The listing builds one solid part. Answer for the finished solid, in the listing's coordinates (mm). Coordinates: 2 decimals unless noted, no trailing zeros. Loops run counter-clockwise (first coordinate to the right, second up) from the corner with the lowest first, then second, coordinate; pieces in that order, holes last. Notation, with made-up numbers: (-29.75, 23) - (3.25, 23) arc R26 cw to (3.25, 52) - close; hole circle Ø2 at (52.25, 40.5). An arc over 180 degrees is marked (long way). One line per question, with ' | ' between items.
from build123d import *

# Parameters (mm, degrees)
F0_R     = 1.5875
F1_DEPTH = 3.048


with BuildPart() as f1:
    # F0 (on Front) → F1 (new body)
    with BuildSketch(Plane.XZ):
        with BuildLine():
            ThreePointArc((-9.5341186691, 52.2447508267), (-6.7171678622, 45.5597172954), (-0.0094340062, 42.7972561321))
            ThreePointArc((-0.0094340062, 42.7972561321), (6.7257580846, 45.5870640413), (9.5155659938, 52.3222561321))
            ThreePointArc((9.5155659938, 52.3222561321), (9.4949130682, 52.9491625761), (9.4330438542, 53.573350395))
            ThreePointArc((9.4330438542, 53.573350395), (0.5455224312, 61.8310756357), (-9.2422673958, 54.6632842395))
            Line((-9.2422673958, 54.6632842395), (-9.5341186691, 52.2447508267))
        make_face()
        with BuildLine():
            ThreePointArc((3.1655659938, 52.3222561321), (2.235630024, 50.0771921018), (-0.0094340062, 49.1472561321))
            ThreePointArc((-0.0094340062, 49.1472561321), (-2.2544980365, 54.5673201623), (3.1655659938, 52.3222561321))
        make_face(mode=Mode.SUBTRACT)
        with BuildLine():
            ThreePointArc((9.5155659938, 52.3222561321), (6.7257580846, 45.5870640413), (-0.0094340062, 42.7972561321))
            Line((-0.0094340062, 42.7972561321), (-0.0094340062, 38.0458299899))
            Line((-0.0094340062, 38.0458299899), (0.1854236079, 17.3965493596))
            ThreePointArc((0.1854236079, 17.3965493596), (10.4432233162, 13.7633317509), (15.9512497798, 4.3780043978))
            Line((15.9512497798, 4.3780043978), (9.4330438542, 53.573350395))
            ThreePointArc((9.4330438542, 53.573350395), (9.4949130682, 52.9491625761), (9.5155659938, 52.3222561321))
        make_face()
        with BuildLine():
            Line((-0.0094340062, 38.0458299899), (-0.0094340062, 42.7972561321))
            ThreePointArc((-0.0094340062, 42.7972561321), (-6.7171678622, 45.5597172954), (-9.5341186691, 52.2447508267))
            Line((-9.5341186691, 52.2447508267), (-15.4254400006, 3.4241398184))
            ThreePointArc((-15.4254400006, 3.4241398184), (-10.3245703873, 13.2859483017), (-0.0094340062, 17.3935143465))
            Line((-0.0094340062, 17.3935143465), (-0.0094340062, 38.0458299899))
        make_face()
        with Locations((-1.6167838335, 40.1418484393)):
            Circle(F0_R, mode=Mode.SUBTRACT)
        with BuildLine():
            ThreePointArc((-9.2422673958, 54.6632842395), (-9.4658311447, 53.4633863439), (-9.5341186691, 52.2447508267))
            Line((-9.5341186691, 52.2447508267), (-9.2422673958, 54.6632842395))
        make_face()
        with BuildLine():
            Line((-0.0094340062, 4.678493973), (-0.0094340062, 17.3935143465))
            ThreePointArc((-0.0094340062, 17.3935143465), (-10.3245703873, 13.2859483017), (-15.4254400006, 3.4241398184))
            ThreePointArc((-15.4254400006, 3.4241398184), (-15.5386299257, 1.7131836533), (-15.4666248709, 0))
            ThreePointArc((-15.4666248709, 0), (-10.4652805135, -10.1123806344), (-0.0094340062, -14.3490020823))
            Line((-0.0094340062, -14.3490020823), (-0.0094340062, -1.6339817089))
            ThreePointArc((-0.0094340062, -1.6339817089), (-2.8397781032, 1.5222561321), (-0.0094340062, 4.678493973))
        make_face()
        with BuildLine():
            ThreePointArc((15.9512497798, 4.3780043978), (10.4432233162, 13.7633317509), (0.1854236079, 17.3965493596))
            Line((0.1854236079, 17.3965493596), (0.305262239, 4.6971147776))
            ThreePointArc((0.305262239, 4.6971147776), (2.5696684822, 3.7778876305), (3.5102218968, 1.5222561321))
            ThreePointArc((3.5102218968, 1.5222561321), (2.4549320784, -0.8415234148), (-0.0094340062, -1.6339817089))
            Line((-0.0094340062, -1.6339817089), (-0.0094340062, -14.3490020823))
            ThreePointArc((-0.0094340062, -14.3490020823), (8.4967936253, -12.09407127), (14.495092683, -5.6550472833))
            ThreePointArc((14.495092683, -5.6550472833), (15.7754870132, -2.1674373693), (16.2102218968, 1.5222561321))
            ThreePointArc((16.2102218968, 1.5222561321), (16.1453463055, 2.9559894332), (15.9512497798, 4.3780043978))
        make_face()
        with BuildLine():
            ThreePointArc((-0.0094340062, -14.3490020823), (-10.4652805135, -10.1123806344), (-15.4666248709, 0))
            Line((-15.4666248709, 0), (-9.5284841955, -61.6411305964))
            ThreePointArc((-9.5284841955, -61.6411305964), (-6.6245448741, -55.1245742942), (-0.0094340062, -52.4527438679))
            Line((-0.0094340062, -52.4527438679), (-0.0094340062, -14.3490020823))
        make_face()
        with BuildLine():
            ThreePointArc((14.495092683, -5.6550472833), (8.4967936253, -12.09407127), (-0.0094340062, -14.3490020823))
            Line((-0.0094340062, -14.3490020823), (-0.0094340062, -52.4527438679))
            ThreePointArc((-0.0094340062, -52.4527438679), (6.7257580846, -55.2425517771), (9.5155659938, -61.9777438679))
            Line((9.5155659938, -61.9777438679), (36.5030659938, -61.9777438679))
            ThreePointArc((36.5030659938, -61.9777438679), (38.9286766306, -56.2660907011), (44.7230299367, -54.0452713422))
            Line((44.7230299367, -54.0452713422), (18.5079615272, -53.1084211888))
            ThreePointArc((18.5079615272, -53.1084211888), (12.8201303591, -50.41150042), (10.8761098535, -44.4243818055))
            Line((10.8761098535, -44.4243818055), (14.495092683, -5.6550472833))
        make_face()
        with BuildLine():
            ThreePointArc((-0.0094340062, -52.4527438679), (-6.6245448741, -55.1245742942), (-9.5284841955, -61.6411305964))
            ThreePointArc((-9.5284841955, -61.6411305964), (-6.8593267813, -68.5962477752), (0, -71.502739196))
            Line((0, -71.502739196), (0.6586396335, -71.4792859855))
            ThreePointArc((0.6586396335, -71.4792859855), (6.9579552616, -68.4724426131), (9.5155659938, -61.9777438679))
            Line((9.5155659938, -61.9777438679), (3.1655659938, -61.9777438679))
            ThreePointArc((3.1655659938, -61.9777438679), (-2.2544980365, -64.2228078982), (-0.0094340062, -58.8027438679))
            Line((-0.0094340062, -58.8027438679), (-0.0094340062, -52.4527438679))
        make_face()
        with BuildLine():
            Line((0.6586396335, -71.4792859855), (0, -71.502739196))
            ThreePointArc((0, -71.502739196), (0.3295227253, -71.4967108988), (0.6586396335, -71.4792859855))
        make_face()
        with BuildLine():
            Line((36.5030659938, -61.9777438679), (9.5155659938, -61.9777438679))
            ThreePointArc((9.5155659938, -61.9777438679), (6.9579552616, -68.4724426131), (0.6586396335, -71.4792859855))
            Line((0.6586396335, -71.4792859855), (44.7230299367, -69.9102163936))
            ThreePointArc((44.7230299367, -69.9102163936), (38.9286766306, -67.6893970348), (36.5030659938, -61.9777438679))
        make_face()
        with BuildLine():
            ThreePointArc((44.7230299367, -54.0452713422), (38.9286766306, -56.2660907011), (36.5030659938, -61.9777438679))
            ThreePointArc((36.5030659938, -61.9777438679), (38.9286766306, -67.6893970348), (44.7230299367, -69.9102163936))
            ThreePointArc((44.7230299367, -69.9102163936), (50.1522191606, -67.4896332311), (52.3780659938, -61.9777438679))
            ThreePointArc((52.3780659938, -61.9777438679), (50.1522191606, -56.4658545048), (44.7230299367, -54.0452713422))
        make_face()
        with BuildLine():
            ThreePointArc((47.6155659938, -61.9777438679), (44.4405659938, -65.1527438679), (41.2655659938, -61.9777438679))
            ThreePointArc((41.2655659938, -61.9777438679), (44.4405659938, -58.8027438679), (47.6155659938, -61.9777438679))
        make_face(mode=Mode.SUBTRACT)
        with BuildLine():
            ThreePointArc((9.5155659938, -61.9777438679), (6.7257580846, -55.2425517771), (-0.0094340062, -52.4527438679))
            Line((-0.0094340062, -52.4527438679), (-0.0094340062, -58.8027438679))
            ThreePointArc((-0.0094340062, -58.8027438679), (2.235630024, -59.7326798377), (3.1655659938, -61.9777438679))
            Line((3.1655659938, -61.9777438679), (9.5155659938, -61.9777438679))
        make_face()
    extrude(amount=F1_DEPTH)


solid = f1.part
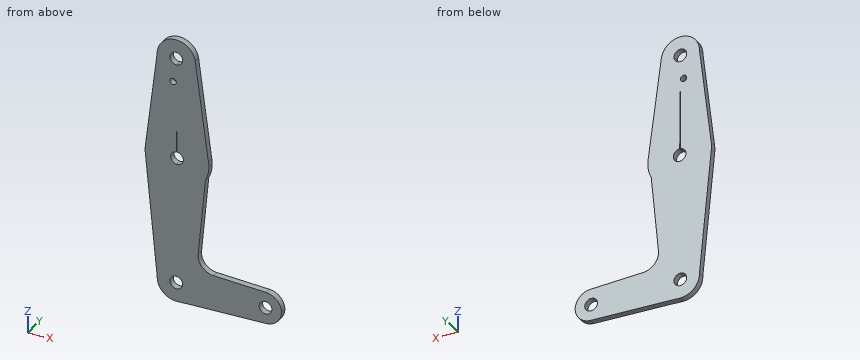
Item 1: Each of these flat-tipped pins is pushed along its axis until it touches: pin 1 Ø3 at (x, z) = (-2.5, -31.5) entering from +Y; pin 2 Ø0.9 at (y, z) = (-2, 24.5) entering from +X. Where does it stop, or does it pass through?
Taken from the geometry:
pin 1: stops at y = 0 | pin 2: stops at x = 13.34
Item 2: Find section B-B, the plane x = 42.5. Write down the section's boundary in (y, z), plus the area to 3 significant figures.
Taken from the geometry:
outline: (-3.05, -69.99) - (0, -69.99) - (0, -64.49) - (-3.05, -64.49) - close; (-3.05, -59.46) - (0, -59.46) - (0, -53.97) - (-3.05, -53.97) - close | area: 33.5 mm2
Item 3: Find section A-A, the plane z = 28. Write down the section's boundary in (x, y), plus the area to 3 significant figures.
Taken from the geometry:
outline: (-12.46, -3.05) - (-0.01, -3.05) - (-0.01, 0) - (-12.46, 0) - close; (0.09, -3.05) - (12.82, -3.05) - (12.82, 0) - (0.09, 0) - close | area: 76.8 mm2
Item 4: Find section C-C, the plane y = -1.5. State how many separate pieces and enclosed holes the cut face has, plus the area to 3 significant figures.
Taken from the geometry:
separate pieces: 1 | enclosed holes: 5 | area: 3,750 mm2
Item 5: Find the intervals of material crossed by line 1 (Z direction, x = -1, y = -0.55); line 2 (Z direction, x = 42.5, y = -0.65); line 3 (Z direction, x = 45.5, y = -0.55), in increasing order. Write a range as [from, to].
Taken from the geometry:
line 1: z = [-71.45, -64.99], [-58.96, -1.36], [4.4, 38.68], [41.6, 49.31], [55.34, 61.8] | line 2: z = [-69.99, -64.49], [-59.46, -53.97] | line 3: z = [-69.84, -64.97], [-58.98, -54.11]
Item 6: Find section D-D, the plane x = 7. Write down the section's boundary in (y, z).
Taken from the geometry:
outline: (-3.05, -71.25) - (0, -71.25) - (0, 58.77) - (-3.05, 58.77) - close
